Design review of the part built by this model. Coordinates are the model's own, in mm. Face numbers are marked on the shaded views. A direction names the side the tool comes from. Round coordinates to 2 decimals unless told otherwise and drop trailing zeros. Loops run counter-clockwise (first coordinate to the right, second up) from the corner with the lowest first, then second, coordinate; pieces in that order, holes last. Notation, with made-up numbers: (-4.75, -18) - (14.25, -18) arc R9 ccw to (14.25, -8) - close; hole circle Ø9 at (-39, 60.5). An arc over 180 degrees is marked (long way). Use one line per item in the form item = value. Start each with the question number.
(1) Machinability: for the marked faces 1 and 2, which of the approach directions +Z, -Z, +X, -X, +Y, -Y give a long, thin tool a straight path to every point of the face, cutting with its end or side? Answer none if there is none.
(2) Wall thickness on probe 1 along Y at (x, z) = (57.15, 14.75); probe 2 along X at (y, z) = (-19.05, 9); probe 3 along X at (y, z) = (-22, 11.5): over which ranges is each line inside the solid? List them lowest first. Write a range as [from, to].
(3) We need section D-D, the plane x = -32.5. Write out the cut boundary in (y, z), then the cut area to 3 significant figures.
(4) For pin 1 (11.5 mm diameter, centred on x = -57.15, y = 19.05, fed in from -Z); pin 2 (3 mm diameter, centred on x = -55, y = 27, fed in from +Z); pin 3 (12 mm diameter, centred on y = -16.5, z = 28, fed in from +X); pin 4 (5 mm diameter, centred on y = -11, z = 34.5, fed in from +X), all flat-tipped, find the tip position at first contact; note any pin that passes through.
(5) We need section C-C, the plane x = 0. Write out the cut boundary in (y, z), then the cut area to 3 significant figures.
(6) We need section B-B, the plane y = 0. Write out the cut boundary in (x, z).
(7) We need section A-A, the plane x = -57.15. Write out the cut boundary in (y, z), then the cut area to 3 significant figures.
from build123d import *

# Parameters (mm, degrees)
F0_W     = 152.4
F0_H     = 76.2
F1_DEPTH = 25.4
F2_R     = 6.35
F3_DEPTH = 25.401
F4_SIZE  = 5.08
F5_W     = 25.4
F5_H     = 50.8
F7_W     = 10.3809926659
F7_H     = 12.2932828963
F9_R     = 2.54
F10_R    = 2.54


with BuildPart() as f1:
    # F0 (on Top) → F1 (new body)
    with BuildSketch(Plane.XY):
        Rectangle(F0_W, F0_H)
    extrude(amount=F1_DEPTH)

    # F2 (on Top) → F3 (cut, through all)
    with BuildSketch(Plane.XY):
        with Locations((-57.15, 19.05)):
            Circle(F2_R)
        with Locations((-57.15, -19.05)):
            Circle(F2_R)
        with Locations((57.15, -19.05)):
            Circle(F2_R)
        with Locations((57.15, 19.05)):
            Circle(F2_R)
    extrude(amount=F3_DEPTH, mode=Mode.SUBTRACT)

    # F4
    f4_edges = [f1.edges().sort_by_distance(p)[0] for p in [
        (0, 38.1, 25.4),
        (76.2, 0, 25.4),
        (-76.2, 0, 25.4),
        (0, -38.1, 25.4),
        (-63.5, -19.05, 25.4),
        (50.8, -19.05, 25.4),
        (-63.5, 19.05, 25.4),
        (50.8, 19.05, 25.4),
    ]]
    chamfer(f4_edges, length=F4_SIZE)

    # F5 (on Front) → F6 (revolve)
    with BuildSketch(Plane.XZ):
        with Locations((12.7, 50.8)):
            Rectangle(F5_W, F5_H)
    revolve(axis=Axis((0, 0, 50.8), (0, 0, 1)))

    # F7 (on Front) → F8 (revolve, cut)
    with BuildSketch(Plane.XZ):
        with Locations((23.6047832295, 49.3830461055)):
            Rectangle(F7_W, F7_H)
    revolve(axis=Axis((0, 0, 25.4), (0, 0, 1)), mode=Mode.SUBTRACT)

    # F9
    f9_edges = [f1.edges().sort_by_distance(p)[0] for p in [
        (25.4, 0, 34.318202),
        (-25.4, 0, 43.236405),
        (-25.4, 0, 25.4),
    ]]
    fillet(f9_edges, radius=F9_R)

    # F10
    f10_edges = [f1.edges().sort_by_distance(p)[0] for p in [
        (-25.4, 0, 76.2),
    ]]
    fillet(f10_edges, radius=F10_R)


solid = f1.part
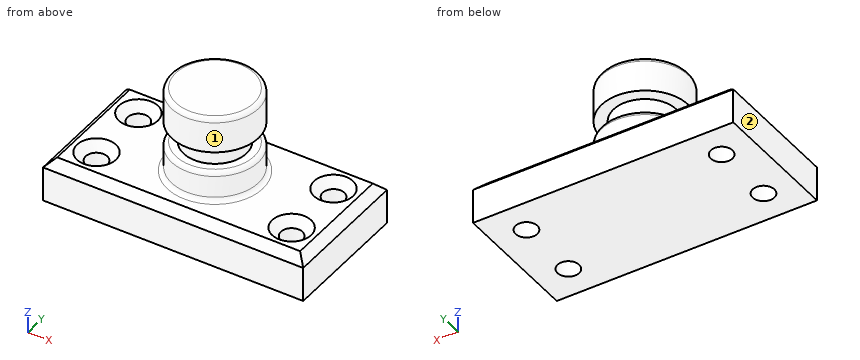
Data:
q1.face_1 = +Z
q1.face_2 = +Z, -Z, -X, +Y, -Y
q2.probe_1 = [-38.1, -25.4], [-12.7, 12.7], [25.4, 38.1]
q2.probe_2 = [-76.2, -63.5], [-50.8, 50.8], [63.5, 76.2]
q2.probe_3 = [-76.2, -62.77], [-51.53, 51.53], [62.77, 76.2]
q3.outline = (-38.1, 0) - (38.1, 0) - (38.1, 20.32) - (33.02, 25.4) - (-33.02, 25.4) - (-38.1, 20.32) - close
q3.area = 1,910 mm^2
q4.pin_1 = through
q4.pin_2 = 23.71
q4.pin_3 = 74.52
q4.pin_4 = 23.94
q5.outline = (-38.1, 0) - (38.1, 0) - (38.1, 20.32) - (33.02, 25.4) - (27.94, 25.4) arc R2.54 cw to (25.4, 27.94) - (25.4, 40.7) arc R2.54 ccw to (22.86, 43.24) - (18.41, 43.24) - (18.41, 55.53) - (25.4, 55.53) - (25.4, 73.66) arc R2.54 ccw to (22.86, 76.2) - (-22.86, 76.2) arc R2.54 ccw to (-25.4, 73.66) - (-25.4, 55.53) - (-18.41, 55.53) - (-18.41, 43.24) - (-22.86, 43.24) arc R2.54 ccw to (-25.4, 40.7) - (-25.4, 27.94) arc R2.54 cw to (-27.94, 25.4) - (-33.02, 25.4) - (-38.1, 20.32) - close
q5.area = 4,320 mm^2
q6.outline = (-76.2, 0) - (76.2, 0) - (76.2, 20.32) - (71.12, 25.4) - (27.94, 25.4) arc R2.54 cw to (25.4, 27.94) - (25.4, 40.7) arc R2.54 ccw to (22.86, 43.24) - (18.41, 43.24) - (18.41, 55.53) - (25.4, 55.53) - (25.4, 73.66) arc R2.54 ccw to (22.86, 76.2) - (-22.86, 76.2) arc R2.54 ccw to (-25.4, 73.66) - (-25.4, 55.53) - (-18.41, 55.53) - (-18.41, 43.24) - (-22.86, 43.24) arc R2.54 ccw to (-25.4, 40.7) - (-25.4, 27.94) arc R2.54 cw to (-27.94, 25.4) - (-71.12, 25.4) - (-76.2, 20.32) - close
q7.outline = (-38.1, 0) - (-25.4, 0) - (-25.4, 20.32) - (-30.48, 25.4) - (-33.02, 25.4) - (-38.1, 20.32) - close; (-12.7, 0) - (12.7, 0) - (12.7, 20.32) - (7.62, 25.4) - (-7.62, 25.4) - (-12.7, 20.32) - close; (25.4, 0) - (38.1, 0) - (38.1, 20.32) - (33.02, 25.4) - (30.48, 25.4) - (25.4, 20.32) - close
q7.area = 1,210 mm^2
